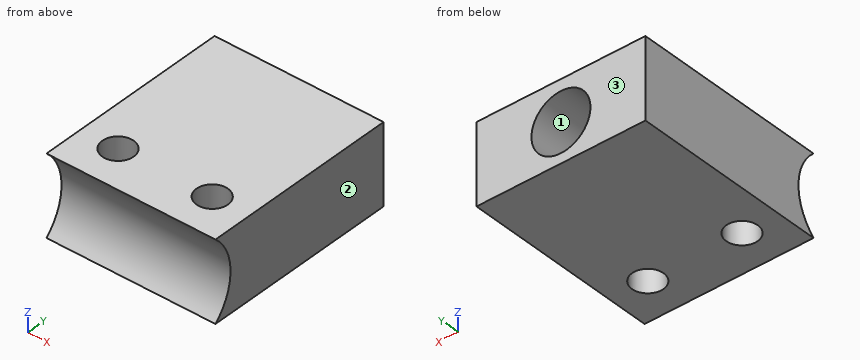
from build123d import *

# Parameters (mm, degrees)
SKETCH1_W           = 21.53
SKETCH1_H           = 30
BOSS_EXTRUDE1_DEPTH = 10.2
SKETCH2_R           = 3.76
CUT_EXTRUDE1_DEPTH  = 10
CUT_EXTRUDE2_REACH  = 30.153
SKETCH3_W           = 10.2
SKETCH3_H           = 4.899707594
CUT_EXTRUDE3_REACH  = 23.093
SKETCH4_R           = 2


with BuildPart() as part:
    # Sketch1 → Boss-Extrude1 (new body)
    with BuildSketch(Plane.XY):
        Rectangle(SKETCH1_W, SKETCH1_H)
    extrude(amount=BOSS_EXTRUDE1_DEPTH)

    # Sketch2 → Cut-Extrude1 (cut)
    with BuildSketch(Plane(origin=(0, 15, 0), x_dir=(1, 0, 0), z_dir=(0, 1, 0))):
        with Locations(Location((0, -5, 0), (0, 0, 270))):
            Circle(SKETCH2_R)
    extrude(amount=-CUT_EXTRUDE1_DEPTH, mode=Mode.SUBTRACT)

    # Sketch3 → Cut-Extrude2 (cut, up to next)
    with BuildSketch(Plane(origin=(10.765, 0, 0), x_dir=(0, 0, -1), z_dir=(1, 0, 0)), mode=Mode.PRIVATE) as cut_extrude2_sk1:
        with BuildLine():
            ThreePointArc((-10.2, -10.100292406), (-5.1, -7.850979668), (0, -10.100292406))
            Line((0, -10.100292406), (-10.2, -10.100292406))
        make_face()
    cut_extrude2_tool1 = extrude(cut_extrude2_sk1.sketch, amount=-CUT_EXTRUDE2_REACH, mode=Mode.PRIVATE) & part.part
    # Sketch3 → Cut-Extrude2 (cut, up to next)
    with BuildSketch(Plane(origin=(10.765, 0, 0), x_dir=(0, 0, -1), z_dir=(1, 0, 0)), mode=Mode.PRIVATE) as cut_extrude2_sk2:
        with Locations((-5.1, -12.550146203)):
            Rectangle(SKETCH3_W, SKETCH3_H)
    cut_extrude2_tool2 = extrude(cut_extrude2_sk2.sketch, amount=-CUT_EXTRUDE2_REACH, mode=Mode.PRIVATE) & part.part
    add(cut_extrude2_tool1.solids().sort_by_distance((10.765, -9.186693, 5.1))[0], mode=Mode.SUBTRACT)
    add(cut_extrude2_tool2.solids().sort_by_distance((10.765, -12.550146, 5.1))[0], mode=Mode.SUBTRACT)

    # Sketch4 → Cut-Extrude3 (cut, up to next)
    with BuildSketch(Plane.XY.offset(10.2), mode=Mode.PRIVATE) as cut_extrude3_sk1:
        with Locations((-6, -5)):
            Circle(SKETCH4_R)
    cut_extrude3_tool1 = extrude(cut_extrude3_sk1.sketch, amount=-CUT_EXTRUDE3_REACH, mode=Mode.PRIVATE) & part.part
    # Sketch4 → Cut-Extrude3 (cut, up to next)
    with BuildSketch(Plane.XY.offset(10.2), mode=Mode.PRIVATE) as cut_extrude3_sk2:
        with Locations((6, -5)):
            Circle(SKETCH4_R)
    cut_extrude3_tool2 = extrude(cut_extrude3_sk2.sketch, amount=-CUT_EXTRUDE3_REACH, mode=Mode.PRIVATE) & part.part
    add(cut_extrude3_tool1.solids().sort_by_distance((-6, -5, 10.2))[0], mode=Mode.SUBTRACT)
    add(cut_extrude3_tool2.solids().sort_by_distance((6, -5, 10.2))[0], mode=Mode.SUBTRACT)


solid = part.part
The listing builds one solid part. Answer for the finished solid, in the listing's coordinates (mm). Face numbers are marked on the shaded views. Give positions to 0.01 mm unless a question says otherwise; leave off trailing zeros. Order: outer loops, then holes, each group sorted by start corner. A loop starts at its lowest first (then second) coordinate and runs counter-clockwise, first axis right, second up. Notation, with made-up numbers: (-37, -14.5) - (9, -14.5) arc R23 cw to (9, 15.5) - close; hole circle Ø9 at (-6, -19). An arc over 180 degrees is marked (long way). Use one line per item in the form item = value.
1) Find section C-C on z = 2. Determine the outline of the cut face in (x, y) (3 decimals), and give its area (3 significant figures).
Verdict:
outline = (-10.765, -8.586) - (10.765, -8.586) - (10.765, 15) - (2.267, 15) - (2.267, 5) - (-2.267, 5) - (-2.267, 15) - (-10.765, 15) - close; hole circle Ø4 at (-6, -5); hole circle Ø4 at (6, -5)
area = 437 mm^2
2) Find section A-A on x = -6. Determine the outline of the cut face in (y, z), and give its area (3 significant figures).
Verdict:
outline = (-10.1, 0) - (-7, 0) - (-7, 10.2) - (-10.1, 10.2) arc R6.91 cw to start; (-3, 0) - (15, 0) - (15, 10.2) - (-3, 10.2) - close
area = 199 mm^2
3) Find section B-B on y = -3.75. Determine the outline of the cut face in (x, z) (3 decimals).
Verdict:
outline = (-10.765, 0) - (-7.561, 0) - (-7.561, 10.2) - (-10.765, 10.2) - close; (-4.439, 0) - (4.439, 0) - (4.439, 10.2) - (-4.439, 10.2) - close; (7.561, 0) - (10.765, 0) - (10.765, 10.2) - (7.561, 10.2) - close
4) This flat-tipped pin is pushed along its axis until it touches: pin 1 (4 mm diameter, centred on x = 1, z = 5.5, fed in from +Y). Where does it stop, or does it pass through?
Verdict:
pin_1 = 5
5) The mould has two halves that part along X. Classify the marked faces 1, 2 and 3: released by +X, released by -X, zero draft, split by the parting line, or undercut.
Verdict:
face_1 = undercut
face_2 = released by +X
face_3 = zero draft
6) Consider probe 1 along X at (y, z) = (12.5, 5) (3 decimals); probe 2 along Z at (x, y) = (2, 11.5); probe 3 along Y at (x, z) = (-6, 5.25). Determine where each line is inside the solid, lowest interval first. Write a range as [from, to].
Verdict:
probe_1 = [-10.765, -3.76], [3.76, 10.765]
probe_2 = [0, 1.82], [8.18, 10.2]
probe_3 = [-7.85, -7], [-3, 15]
7) Find section D-D on y = 9. Determine the outline of the cut face in (x, z) (3 decimals).
Verdict:
outline = (-10.765, 0) - (10.765, 0) - (10.765, 10.2) - (-10.765, 10.2) - close; hole circle Ø7.52 at (0, 5)
